Build history of the part. All positions in model axes, mm. A direction names the side the tool comes from. Round coordinates to 2 decimals unless told otherwise and drop trailing zeros. Order: outer loops, then holes, each group sorted by start corner. A loop starts at its lowest first (then second) coordinate and runs counter-clockwise, first axis right, second up. Notation, with made-up numbers: (23.25, 80.25) -> (27.25, 80.25) arc R10 ccw to (27.25, 95.25) -> close; hole circle Ø1 at (66.25, -33). An arc over 180 degrees is marked (long way). Answer as a JSON object with one key per item and string values.
from build123d import *

# Parameters (mm, degrees)
SKETCH2_W                        = 127
SKETCH2_H                        = 127
HOUSING_DEPTH                    = 39.5
SKETCH4_OUTSIDE_W                = 165.78
SKETCH4_OUTSIDE_H                = 165.78
SKETCH4_OUTSIDE_R                = 45.974
CUT_EXTRUDE2_DEPTH               = 4.698
MOUNTING_POCKETS_DEPTH           = 24.384
ENG_METRIC_SLOT_VERTICAL_REACH   = 160.723
ENG_METRIC_SLOT_HORIZONTAL_DEPTH = 199.381065075
FILLET3_R                        = 0.508
SKETCH213_W                      = 57.15
SKETCH213_H                      = 57.15
EXTRUDE1_DEPTH                   = 26.924
SKETCH214_R                      = 23.8125
CUT_EXTRUDE3_DEPTH               = 5
SKETCH215_R                      = 3.175
CUT_EXTRUDE4_DEPTH               = 21.924
CUT_EXTRUDE5_REACH               = 170.363
SKETCH216_W                      = 42.545
SKETCH216_H                      = 3.048
F_8_32_TAPPED_HOLE1_D            = 3.4544
F_8_32_TAPPED_HOLE1_DEPTH        = 10.7086
F_8_32_TAPPED_HOLE1_TIP          = 1.037806461
SKETCH241_R                      = 45.974
CUT_EXTRUDE7_DEPTH               = 4.698
SKETCH3_R                        = 19.05
CUT_EXTRUDE8_DEPTH               = 122.723587102


with BuildPart() as part:
    # Sketch2 → HOUSING (new body)
    with BuildSketch(Plane.XY):
        Rectangle(SKETCH2_W, SKETCH2_H)
    extrude(amount=HOUSING_DEPTH)

    # Sketch4 outside → Cut-Extrude2 (cut)
    with BuildSketch(Plane.XY.offset(39.5)):
        Rectangle(SKETCH4_OUTSIDE_W, SKETCH4_OUTSIDE_H)
        Circle(SKETCH4_OUTSIDE_R, mode=Mode.SUBTRACT)
    extrude(amount=-CUT_EXTRUDE2_DEPTH, mode=Mode.SUBTRACT)

    # Sketch8 → MOUNTING POCKETS (cut)
    with BuildSketch(Plane.XY.offset(34.802)):
        with BuildLine():
            Line((3.048, -63.5), (3.048, -57.528018122))
            ThreePointArc((3.048, -57.528018122), (4.194729662, -53.888172274), (7.220748912, -51.562946647))
            Line((7.220748912, -51.562946647), (45.320748912, -37.656446647))
            ThreePointArc((45.320748912, -37.656446647), (51.137845848, -38.418247784), (53.848, -43.621518122))
            Line((53.848, -43.621518122), (53.848, -63.5))
            Line((53.848, -63.5), (3.048, -63.5))
        make_face()
        with BuildLine():
            Line((3.048, 63.5), (53.848, 63.5))
            Line((53.848, 63.5), (53.848, 43.621518122))
            ThreePointArc((53.848, 43.621518122), (51.137845848, 38.418247784), (45.320748912, 37.656446647))
            Line((45.320748912, 37.656446647), (7.220748912, 51.562946647))
            ThreePointArc((7.220748912, 51.562946647), (4.194729662, 53.888172274), (3.048, 57.528018122))
            Line((3.048, 57.528018122), (3.048, 63.5))
        make_face()
    extrude(amount=-MOUNTING_POCKETS_DEPTH, mode=Mode.SUBTRACT)

    # Sketch21 → ENG_METRIC SLOT VERTICAL (cut, up to next)
    with BuildSketch(Plane(origin=(63.5, -23.646142673, 1.166551585), x_dir=(0, 0, -1), z_dir=(1, 0, 0)), mode=Mode.PRIVATE) as eng_metric_slot_vertical_sk1:
        with BuildLine():
            Line((-20.641506099, 75.242113831), (-21.041506099, 76.042113831))
            ThreePointArc((-21.041506099, 76.042113831), (-25.829419573, 77.63808499), (-27.425390732, 72.850171515))
            Line((-27.425390732, 72.850171515), (-27.025390732, 72.050171515))
            ThreePointArc((-27.025390732, 72.050171515), (-22.237477257, 70.454200357), (-20.641506099, 75.242113831))
        make_face()
    eng_metric_slot_vertical_tool1 = extrude(eng_metric_slot_vertical_sk1.sketch, amount=-ENG_METRIC_SLOT_VERTICAL_REACH, mode=Mode.PRIVATE) & part.part
    # Sketch21 → ENG_METRIC SLOT VERTICAL (cut, up to next)
    with BuildSketch(Plane(origin=(63.5, -23.646142673, 1.166551585), x_dir=(0, 0, -1), z_dir=(1, 0, 0)), mode=Mode.PRIVATE) as eng_metric_slot_vertical_sk2:
        with BuildLine():
            Line((-27.025390732, -24.757886169), (-27.425390732, -25.557886169))
            ThreePointArc((-27.425390732, -25.557886169), (-25.829419573, -30.345799643), (-21.041506099, -28.749828485))
            Line((-21.041506099, -28.749828485), (-20.641506099, -27.949828485))
            ThreePointArc((-20.641506099, -27.949828485), (-22.237477257, -23.16191501), (-27.025390732, -24.757886169))
        make_face()
    eng_metric_slot_vertical_tool2 = extrude(eng_metric_slot_vertical_sk2.sketch, amount=-ENG_METRIC_SLOT_VERTICAL_REACH, mode=Mode.PRIVATE) & part.part
    add(eng_metric_slot_vertical_tool1.solids().sort_by_distance((63.5, 50.4, 25.2))[0], mode=Mode.SUBTRACT)
    add(eng_metric_slot_vertical_tool2.solids().sort_by_distance((63.5, -50.4, 25.2))[0], mode=Mode.SUBTRACT)

    # Sketch212 → ENG_METRIC SLOT HORIZONTAL (cut, through all)
    with BuildSketch(Plane(origin=(34.062086582, -104.655987826, 0), x_dir=(-1, 0, 0), z_dir=(0, 0, -1))):
        with BuildLine():
            Line((12.254028899, 156.251958985), (11.854028899, 157.051958985))
            ThreePointArc((11.854028899, 157.051958985), (7.066115424, 158.647930143), (5.470144266, 153.860016668))
            Line((5.470144266, 153.860016668), (5.870144266, 153.060016668))
            ThreePointArc((5.870144266, 153.060016668), (10.658057741, 151.46404551), (12.254028899, 156.251958985))
        make_face()
        with BuildLine():
            Line((5.870144266, 56.251958985), (5.470144266, 55.451958985))
            ThreePointArc((5.470144266, 55.451958985), (7.066115424, 50.66404551), (11.854028899, 52.260016668))
            Line((11.854028899, 52.260016668), (12.254028899, 53.060016668))
            ThreePointArc((12.254028899, 53.060016668), (10.658057741, 57.847930143), (5.870144266, 56.251958985))
        make_face()
    extrude(amount=-ENG_METRIC_SLOT_HORIZONTAL_DEPTH, mode=Mode.SUBTRACT)

    # Fillet3
    fillet3_edges = [part.edges().sort_by_distance(p)[0] for p in [
        (3.048, -60.514009061, 10.418),
        (4.194729662, -53.888172274, 10.418),
        (26.270748912, -44.609696647, 10.418),
        (51.137845848, -38.418247784, 10.418),
        (53.848, -53.560759061, 10.418),
        (51.137845848, 38.418247784, 10.418),
        (26.270748912, 44.609696647, 10.418),
        (4.194729662, 53.888172274, 10.418),
        (3.048, 60.514009061, 10.418),
        (53.848, 53.560759061, 10.418),
    ]]
    fillet(fillet3_edges, radius=FILLET3_R)

    # Sketch213 → Extrude1 (add)
    with BuildSketch(Plane.XZ.offset(63.5)):
        with Locations((-37.084, 30.48)):
            Rectangle(SKETCH213_W, SKETCH213_H)
    extrude(amount=EXTRUDE1_DEPTH)

    # Sketch214 → Cut-Extrude3 (cut)
    with BuildSketch(Plane.XZ.offset(90.424)):
        with Locations(Location((-37.084, 30.48, 0), (0, 0, 270))):
            Circle(SKETCH214_R)
    extrude(amount=-CUT_EXTRUDE3_DEPTH, mode=Mode.SUBTRACT)

    # Sketch215 → Cut-Extrude4 (cut)
    with BuildSketch(Plane.XZ.offset(85.424)):
        with Locations(Location((-37.084, 30.48, 0), (0, 0, 270))):
            Circle(SKETCH215_R)
    extrude(amount=-CUT_EXTRUDE4_DEPTH, mode=Mode.SUBTRACT)

    # Sketch216 → Cut-Extrude5 (cut, up to next)
    with BuildSketch(Plane.ZY.offset(65.659), mode=Mode.PRIVATE) as cut_extrude5_sk1:
        with Locations((37.7825, -65.024)):
            Rectangle(SKETCH216_W, SKETCH216_H)
    cut_extrude5_tool1 = extrude(cut_extrude5_sk1.sketch, amount=-CUT_EXTRUDE5_REACH, mode=Mode.PRIVATE) & part.part
    add(cut_extrude5_tool1.solids().sort_by_distance((-65.659, -65.024, 37.7825))[0], mode=Mode.SUBTRACT)

    # #8-32 Tapped Hole1
    with Locations(Plane.XZ.offset(90.424)):
        with Locations((-60.706, 6.858), (-60.706, 54.102), (-13.462, 54.102), (-13.462, 6.858)):
            Hole(F_8_32_TAPPED_HOLE1_D / 2, depth=F_8_32_TAPPED_HOLE1_DEPTH)
            with Locations((0, 0, -(F_8_32_TAPPED_HOLE1_DEPTH + F_8_32_TAPPED_HOLE1_TIP / 2))):  # 118° drill point
                Cone(0, F_8_32_TAPPED_HOLE1_D / 2, F_8_32_TAPPED_HOLE1_TIP, mode=Mode.SUBTRACT)

    # Sketch241 → Cut-Extrude7 (cut)
    with BuildSketch(Plane.XY.offset(39.5)):
        Circle(SKETCH241_R)
    extrude(amount=-CUT_EXTRUDE7_DEPTH, mode=Mode.SUBTRACT)

    # Sketch3 → Cut-Extrude8 (cut, through all)
    with BuildSketch(Plane.XY.offset(48.26)):
        Circle(SKETCH3_R)
    extrude(amount=-CUT_EXTRUDE8_DEPTH, mode=Mode.SUBTRACT)


solid = part.part
1) Cut at B-B, the plane y = 12.5. Give the cut face in (x, z).
Checked values:
{"outline": "(-63.5, 0) -> (-14.38, 0) -> (-14.38, 34.8) -> (-63.5, 34.8) -> close; (14.38, 0) -> (63.5, 0) -> (63.5, 34.8) -> (14.38, 34.8) -> close"}
2) Which spindle directions (+Z, -Z, +X, -X, +Y, -Y) get a long thin tool onto all of the face, cutting with end or side? Do faces 4 (the face through (34, -53, 10.418)), 5 (the face through (-13.474, -87.959, 33.58)), 6 (the face through (3.048, 60, 23)). Say none if no direction does.
Checked values:
{"face 4": "+Z, -Y", "face 5": "-Y", "face 6": "+Z, +Y"}
3) Cut at A-A, the plane z = 25.4. Count the separate pieces of the cut face and the enclosed holes in it, plus the area to 3 significant figures.
Checked values:
{"separate pieces": "4", "enclosed holes": "1", "area": "14,000 mm²"}
4) Flat gauge pins, fed straight in: pin 1 Ø6 at (y, z) = (49, 21) entering from -X; pin 2 Ø20.5 at (x, y) = (35, -55) entering from +Z; pin 3 Ø6 at (y, z) = (-72, 34.5) entering from +X. Where does each tip first touch, or does it go through?
Checked values:
{"pin 1": "stops at x = -63.5", "pin 2": "stops at z = 10.42", "pin 3": "stops at x = -8.51"}
5) Cut at D-D, the plane z = 47. Give the cut face in (x, y).
Checked values:
{"outline": "(-65.66, -90.42) -> (-54.23, -90.42) -> (-54.23, -85.42) -> (-19.93, -85.42) -> (-19.93, -90.42) -> (-8.51, -90.42) -> (-8.51, -66.55) -> (-65.66, -66.55) -> close"}
6) Pull direction X, two halves, no side cores. Call faces 1 (the face through (-15, 15, 0)), 2 (the face through (-13.18, -78.86, 6.74)), 3 (the face through (63.5, -1, 17)): pulls with the +X half, pulls with the -X half, needs draft (parallel to the pull), parting line crosses it, or undercut.
Checked values:
{"face 1": "needs draft", "face 2": "undercut", "face 3": "pulls with the +X half"}
7) Probe L1, parallel to X at y = -76, z = 31; L2, parallel to Y at x = 1, z = 18; L3, parallel to X at y = -78.75, z = 30.48. List the from-to ranges inside material, lowest first. Write a range as from..to.
Checked values:
{"L1": "x = -65.66..-40.22, -33.95..-8.51", "L2": "y = -63.5..-19.02, 19.02..63.5", "L3": "x = -65.66..-40.26, -33.91..-8.51"}
8) Cut at C-C, the plane x = -43.5. Give the cut face in (y, z) (3 decimals).
Checked values:
{"outline": "(-90.424, 1.905) -> (-63.5, 1.905) -> (-63.5, 0) -> (63.5, 0) -> (63.5, 34.802) -> (-63.5, 34.802) -> (-63.5, 16.51) -> (-66.548, 16.51) -> (-66.548, 59.055) -> (-90.424, 59.055) -> (-90.424, 53.412) -> (-85.424, 53.412) -> (-85.424, 7.548) -> (-90.424, 7.548) -> close"}
